Build history of the part. All positions in model axes, mm. Face numbers are marked on the shaded views. A direction names the side the tool comes from. Coordinates: 2 decimals unless noted, no trailing zeros. Loops run counter-clockwise (first coordinate to the right, second up) from the corner with the lowest first, then second, coordinate; pieces in that order, holes last.
Item 1: Flat gauge pins, fed straight in: pin 1 (1.5 mm diameter, centred on y = 21.5, z = 22.5, fed in from +X); pin 2 (5.5 mm diameter, centred on x = -30.5, z = 21.5, fed in from +Y). Where does each tip first touch, or does it go through?
Item 2: Cut at D-D (x = -29.5). List the corners of the cut face in (y, z).
Item 3: 3-axis set-ups, long thin cutter, end or side, ignore diameter. For the marked faces 1 and 2: which of +Z, -Z, +X, -X, +Y, -Y reach the whole face in a straight line?
Item 4: Cut at C-C (z = 13.5). List the corners of the cut face in (x, y), and give its area (3 significant figures).
Item 5: Cut at B-B (x = 29.5). List the corners of the cut face in (y, z).
Item 6: Mould opens along Y. For the marked faces 3, 4 and 5 say: released by +Y, released by -Y, zero draft, split by the parting line, or undercut.
Item 7: Cut at A-A (y = 16.5). List the corners of the cut face in (x, z), and give its area (3 significant figures).
Item 8: Drill centre lines: line 1 along Z through (x, y) = (40, 19.5); line 2 along Y through (x, z) = (43, 12); line 3 along X through (y, z) = (17, 20.5). Where is each one in solid material? Low to high.
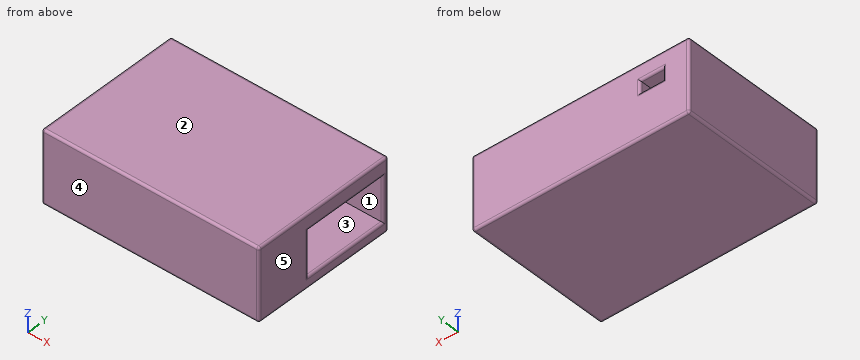
from build123d import *

# Parameters (mm, degrees)
SKETCH1_W           = 93
SKETCH1_H           = 63
BOSS_EXTRUDE1_DEPTH = 31
SKETCH2_W           = 19
SKETCH2_H           = 36.5
CUT_EXTRUDE1_DEPTH  = 31
SKETCH3_W           = 10
SKETCH3_H           = 5
CUT_EXTRUDE2_DEPTH  = 31
FILLET1_R           = 1


with BuildPart() as part:
    # Sketch1 → Boss-Extrude1 (new body)
    with BuildSketch(Plane.XY):
        Rectangle(SKETCH1_W, SKETCH1_H)
    extrude(amount=BOSS_EXTRUDE1_DEPTH)

    # Sketch2 → Cut-Extrude1 (cut)
    with BuildSketch(Plane(origin=(46.5, 0, 0), x_dir=(0, 0, -1), z_dir=(1, 0, 0))):
        with Locations((-14.5, 10.75)):
            Rectangle(SKETCH2_W, SKETCH2_H)
    extrude(amount=-CUT_EXTRUDE1_DEPTH, mode=Mode.SUBTRACT)

    # Sketch3 → Cut-Extrude2 (cut)
    with BuildSketch(Plane(origin=(0, 31.5, 0), x_dir=(1, 0, 0), z_dir=(0, 1, 0))):
        with Locations((-30.5, -21.5)):
            Rectangle(SKETCH3_W, SKETCH3_H)
    extrude(amount=-CUT_EXTRUDE2_DEPTH, mode=Mode.SUBTRACT)

    # Fillet1
    fillet1_edges = [part.edges().sort_by_distance(p)[0] for p in [
        (-46.5, 0, 31),
        (0, -31.5, 31),
        (46.5, 10.75, 24),
        (46.5, -7.5, 14.5),
        (46.5, 10.75, 5),
        (46.5, 29, 14.5),
        (-35.5, 31.5, 21.5),
        (-30.5, 31.5, 24),
        (-25.5, 31.5, 21.5),
        (-30.5, 31.5, 19),
        (46.5, 0, 31),
        (0, -31.5, 0),
        (-46.5, 0, 0),
        (0, 31.5, 0),
        (46.5, 0, 0),
        (46.5, -31.5, 15.5),
        (-46.5, -31.5, 15.5),
        (-46.5, 31.5, 15.5),
        (46.5, 31.5, 15.5),
        (0, 31.5, 31),
    ]]
    fillet(fillet1_edges, radius=FILLET1_R)


solid = part.part
Filled sheet:
1. pin 1: stops at x = 15.5
1. pin 2: stops at y = 31.16
2. outline: (-31.5, 1) arc R1 ccw to (-30.5, 0) - (30.5, 0) arc R1 ccw to (31.5, 1) - (31.5, 18) arc R1 ccw to (30.5, 19) - (0.5, 19) - (0.5, 24) - (30.5, 24) arc R1 ccw to (31.5, 25) - (31.5, 30) arc R1 ccw to (30.5, 31) - (-30.5, 31) arc R1 ccw to (-31.5, 30) - close
3. face 1: +X
3. face 2: +Z, +X, -X, +Y, -Y
4. outline: (-46.5, -30.5) arc R1 ccw to (-45.5, -31.5) - (45.5, -31.5) arc R1 ccw to (46.5, -30.5) - (46.5, -8.5) arc R1 ccw to (45.5, -7.5) - (15.5, -7.5) - (15.5, 29) - (45.5, 29) arc R1 ccw to (46.5, 30) - (46.5, 30.5) arc R1 ccw to (45.5, 31.5) - (-45.5, 31.5) arc R1 ccw to (-46.5, 30.5) - close
4. area: 4,730 mm2
5. outline: (-31.5, 1) arc R1 ccw to (-30.5, 0) - (30.5, 0) arc R1 ccw to (31.5, 1) - (31.5, 30) arc R1 ccw to (30.5, 31) - (-30.5, 31) arc R1 ccw to (-31.5, 30) - close; hole (-7.5, 5) - (29, 5) - (29, 24) - (-7.5, 24) - close
6. face 3: undercut
6. face 4: released by -Y
6. face 5: zero draft
7. outline: (-46.5, 1) arc R1 ccw to (-45.5, 0) - (45.5, 0) arc R1 ccw to (46.5, 1) - (46.5, 4) arc R1 ccw to (45.5, 5) - (15.5, 5) - (15.5, 24) - (45.5, 24) arc R1 ccw to (46.5, 25) - (46.5, 30) arc R1 ccw to (45.5, 31) - (-45.5, 31) arc R1 ccw to (-46.5, 30) - close; hole (-35.5, 19) - (-25.5, 19) - (-25.5, 24) - (-35.5, 24) - close
7. area: 2,240 mm2
8. line 1: z = 0 to 5, 24 to 31
8. line 2: y = -31.5 to -7.5, 29 to 31.5
8. line 3: x = -46.5 to -35.5, -25.5 to 15.5
